Can you work these out from the drawing? Everything is in mm from the part's minimum corner. Round coordinates to 2 decimals unless told otherwise and drop trailing zeros. Order: outer loops, then holes, each group sorted by start corner. A loop starts at its lowest first (then second) coordinate and runs counter-clockwise, first axis right, second up. Notation, with made-up numbers: (-9, 59) - (39, 59) arc R30 cw to (39, 92) - close; hole circle Ø2 at (38.5, 19). An arc over 180 degrees is marked (long way). Write item = value, one per line.
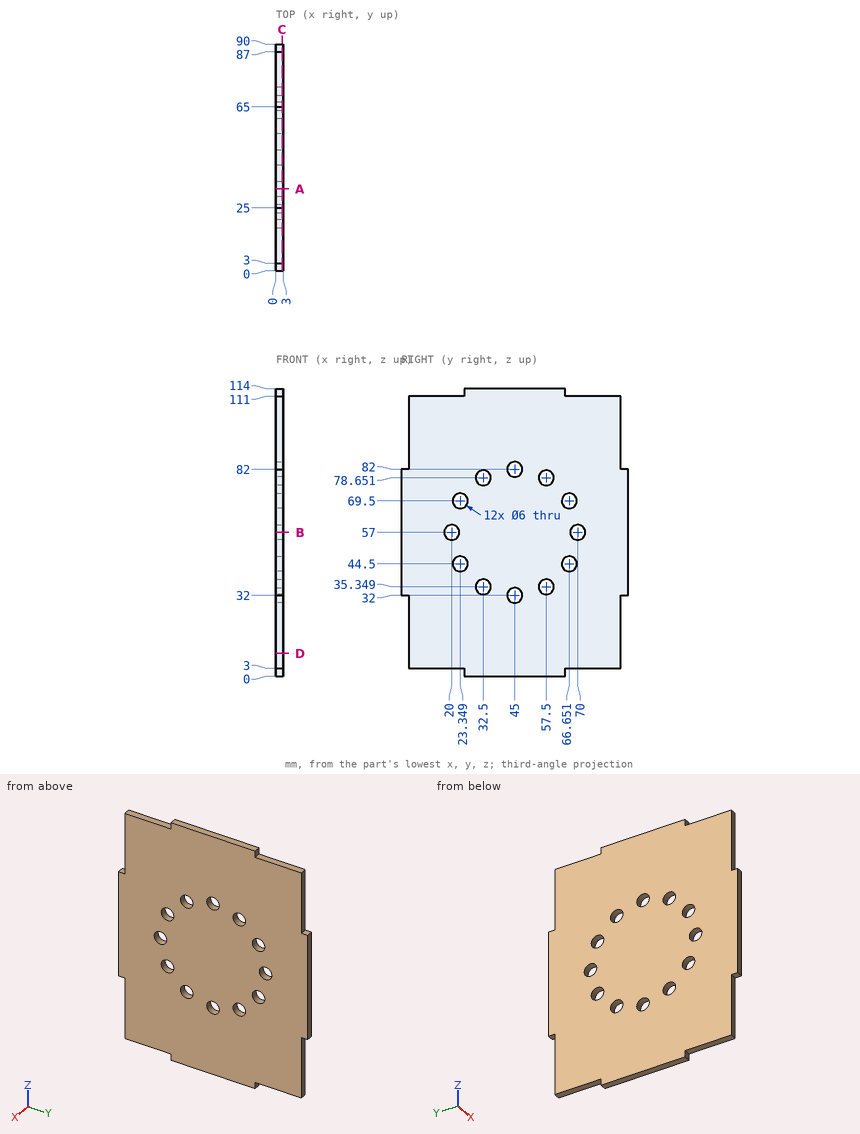
(1) If we section it at C-C (x = 2.45): State how many separate pieces and enclosed holes the cut face has, plus the area to 3 significant figures.
Computed:
separate_pieces = 1
enclosed_holes = 12
area = 9,270 mm^2
(2) If I drill on line 1 (Y direction, x = 1.05, z = 57); line 2 (Y direction, x = 0.3, z = 81) (1 decimal); line 3 (Y direction, x = 2.75, z = 77) (1 decimal), over which ranges is the centre line in solid material (lowest first)? Write a range as from..to.
Computed:
line_1 = 0..17, 23..67, 73..90
line_2 = 0..30.6, 34.4..42.2, 47.8..55.6, 59.4..90
line_3 = 0..30, 35..55, 60..90
(3) Will these pins go through, and if not, where does the flat tip stop? P1, Ø0.9, axis at x = 1, z = 1.5, coming from the -Y side; P2, Ø0.9, axis at x = 2, y = 88, coming from the -Z side; P3, Ø1.5, axis at x = 2, z = 88.5, coming from the -Y side.
Computed:
P1 = 25
P2 = 32
P3 = 3
(4) If we section it at B-B (z = 57): Write out the boundary of the cut face in (x, y), plus the area to 3 significant figures.
Computed:
outline = (0, 0) - (3, 0) - (3, 17) - (0, 17) - close; (0, 23) - (3, 23) - (3, 67) - (0, 67) - close; (0, 73) - (3, 73) - (3, 90) - (0, 90) - close
area = 234 mm^2
(5) If we section it at D-D (z = 9): Write out the boundary of the cut face in (x, y), plus the area to 3 significant figures.
Computed:
outline = (0, 3) - (3, 3) - (3, 87) - (0, 87) - close
area = 252 mm^2
(6) If we section it at A-A (y = 32.5): Write out the boundary of the cut face in (x, z).
Computed:
outline = (0, 0) - (3, 0) - (3, 32.35) - (0, 32.35) - close; (0, 38.35) - (3, 38.35) - (3, 75.65) - (0, 75.65) - close; (0, 81.65) - (3, 81.65) - (3, 114) - (0, 114) - close
